from build123d import *

# Parameters (mm, degrees)
SKETCH_R        = 2.1
PAD_DEPTH       = 7
SKETCH001_R     = 2.25
POCKET_DEPTH    = 22.001
POCKET001_DEPTH = 3.5
SKETCH003_R     = 4.3
POCKET002_DEPTH = 5
SKETCH004_R     = 62
SKETCH004_R_2   = 56
POCKET003_DEPTH = 14.001
CHAMFER_SIZE2   = 3
CHAMFER_SIZE    = 5
FILLET_R        = 2.5
FILLET001_R     = 0.5
POCKET004_DEPTH = 4
SKETCH006_R     = 2.1
PAD001_DEPTH    = 0.2


with BuildPart() as part:
    # Sketch → Pad (new body, symmetric)
    with BuildSketch(Plane.XY):
        with BuildLine():
            Line((-8.5, 20), (-8.5, -20))
            Line((-8.5, -20), (5.5, -20))
            Line((5.5, -20), (5.5, -4))
            Line((5.5, -4), (3.887632, -0.941445))
            ThreePointArc((3.538431, 1.865343), (-3.969398, -0.493844), (3.887632, -0.941445))
            Line((6.5, -3.752556), (3.538431, 1.865343))
            Line((6.5, -15), (6.5, -3.752556))
            Line((13.5, -15), (6.5, -15))
            Line((13.5, -2), (13.5, -15))
            Line((5.5, 13.175467), (13.5, -2))
            Line((5.5, 20), (5.5, 13.175467))
            Line((-8.5, 20), (5.5, 20))
        make_face()
        with Locations((0, 14)):
            Circle(SKETCH_R, mode=Mode.SUBTRACT)
        with Locations((0, -14)):
            Circle(SKETCH_R, mode=Mode.SUBTRACT)
    extrude(amount=PAD_DEPTH, both=True)

    # Sketch001 (on Face10 of Pad) → Pocket (cut, through all)
    with BuildSketch(Plane.YZ.offset(13.5)):
        with Locations((-8, 0)):
            Circle(SKETCH001_R)
    extrude(amount=-POCKET_DEPTH, mode=Mode.SUBTRACT)

    # Sketch002 (on Face15 of Pocket) → Pocket001 (cut)
    with BuildSketch(Plane.YZ.offset(13.5)):
        Polygon((-4.5, 2.020726), (-8, 4.041452), (-11.5, 2.020726), (-11.5, -2.020726), (-8, -4.041452), (-4.5, -2.020726), align=None)
    extrude(amount=-POCKET001_DEPTH, mode=Mode.SUBTRACT)

    # Sketch003 (on Face2 of Pocket001) → Pocket002 (cut)
    with BuildSketch(Plane(origin=(-8.5, 0, 0), x_dir=(0, -1, 0), z_dir=(-1, 0, 0))):
        with Locations((8, 0)):
            Circle(SKETCH003_R)
    extrude(amount=-POCKET002_DEPTH, mode=Mode.SUBTRACT)

    # Sketch004 (on Face5 of Pocket002) → Pocket003 (cut, through all)
    with BuildSketch(Plane.XY.offset(7)):
        with Locations((47.5, 0)):
            Circle(SKETCH004_R)
        with Locations((47.5, 0)):
            Circle(SKETCH004_R_2, mode=Mode.SUBTRACT)
    extrude(amount=-POCKET003_DEPTH, mode=Mode.SUBTRACT)

    # Chamfer
    chamfer_edges = [part.edges().sort_by_distance(p)[0] for p in [
        (5.5, -20, 0),
    ]]
    chamfer_side = part.faces().sort_by_distance((5.5, -12.305712, 0))[0]
    chamfer(chamfer_edges, length=CHAMFER_SIZE, length2=CHAMFER_SIZE2, reference=chamfer_side)

    # Fillet
    fillet_edges = [part.edges().sort_by_distance(p)[0] for p in [
        (2.5, -20, 0),
        (-4.806787, -20, 0),
        (13.5, -15, 0),
        (5.5, 20, 0),
        (13.5, -2, 0),
        (5.5, 13.175467, 0),
        (-4.806787, 20, 0),
    ]]
    fillet(fillet_edges, radius=FILLET_R)

    # Fillet001
    fillet001_edges = [part.edges().sort_by_distance(p)[0] for p in [
        (3.887632, -0.941445, 0),
    ]]
    fillet(fillet001_edges, radius=FILLET001_R)

    # Sketch005 (on Face1 of Fillet001) → Pocket004 (cut)
    with BuildSketch(Plane(origin=(0, 0, -7), x_dir=(1, 0, 0), z_dir=(0, 0, -1))):
        Polygon((4.041452, 14), (2.020726, 17.5), (-2.020726, 17.5), (-4.041452, 14), (-2.020726, 10.5), (2.020726, 10.5), align=None)
        Polygon((4.041452, -14), (2.020726, -10.5), (-2.020726, -10.5), (-4.041452, -14), (-2.020726, -17.5), (2.020726, -17.5), align=None)
    pocket004 = extrude(amount=-POCKET004_DEPTH, mode=Mode.SUBTRACT)

    # Mirrored: Pocket004 across XY
    add(pocket004.mirror(Plane.XY), mode=Mode.SUBTRACT)

    # Sketch006 (on Face46 of Mirrored) → Pad001 (join)
    with BuildSketch(Plane(origin=(0, 0, -3), x_dir=(1, 0, 0), z_dir=(0, 0, -1))):
        with Locations((0, 14)):
            Circle(SKETCH006_R)
        with Locations((0, -14)):
            Circle(SKETCH006_R)
    extrude(amount=-PAD001_DEPTH)


solid = part.part
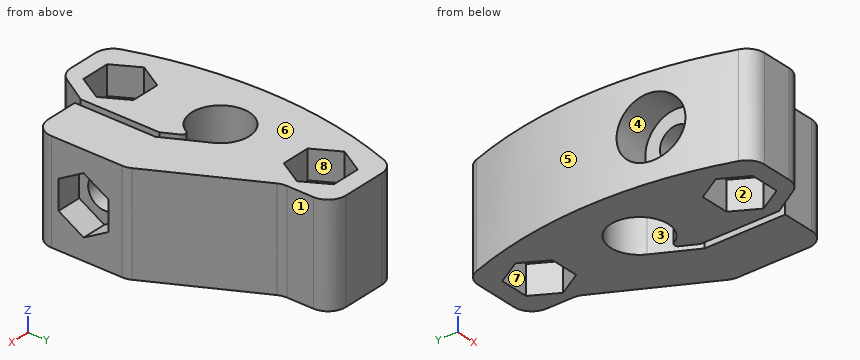
Geometry check sheet. Reference: the model listing, model coordinates, mm. Face numbers are marked on the shaded views. A direction names the side the tool comes from. Coordinates: 2 decimals unless noted, no trailing zeros. Order: outer loops, then holes, each group sorted by start corner. A loop starts at its lowest first (then second) coordinate and runs counter-clockwise, first axis right, second up. Notation, with made-up numbers: (69.25, -24.5) - (108.25, -24.5) arc R26 ccw to (108.25, 3.5) - close; hole circle Ø2 at (-30.75, -3). An arc over 180 degrees is marked (long way). Answer in a Markdown table with one row per item. Add a question column.
1) Set-up check for the marked faces 1, 2, 3 and 4: record each of +Z, -Z, +X, -X, +Y, -Y from which the full face is reachable in a straight line by a thin tool's end or side.
2) Cross-section at B-B, the plane y = 0. Record the cut outline in (x, z), then the cut area to 3 significant figures.
3) Gauge pin test, flat ends, axial feed: P1, Ø5, axis at x = -6, z = 1.5, coming from the +Y side; P2, Ø3.5, axis at x = 0.5, y = -14.5, coming from the -Z side; P3, Ø10.5, axis at x = 0, y = 0, coming from the +Z side; P4, Ø6, axis at x = 9, z = 2, coming from the +Y side. Record the tip position at first contact, or that the pin passes through.
4) Cross-section at A-A, the plane x = 0. State how many separate pieces and enclosed holes the cut face has, then the cut area to 3 significant figures.
5) Cross-section at D-D, the plane x = 7.5. Record the cut outline in (y, z), then the cut area to 3 significant figures.
6) Material ranges on line 1 along Z through (x, y) = (8.4, -8); line 2 along X through (y, z) = (-13.5, -5); line 3 along Y through (x, z) = (0, -1.45), recorded low to high. Write a range as [from, to].
7) Release check for a two-part mould opening along X. For the marked faces 5, 6, 7 and 8 record: +X half, -X half, draft (parallel to the pull), parting line (faces both ways), or undercut.
Check result:
| question | item | result |
|---|---|---|
| 1 | face 1 | +Z, -Z, +X, +Y |
| 1 | face 2 | -Z |
| 1 | face 3 | +Z, -Z |
| 1 | face 4 | -X |
| 2 | outline | (-8.5, -7) - (-4, -7) - (-4, 7) - (-8.5, 7) - close; (4.52, -7) - (12.45, -7) - (12.45, 7) - (4.52, 7) - close |
| 2 | area | 174 mm² |
| 3 | P1 | stops at y = 19.96 |
| 3 | P2 | stops at z = -3 |
| 3 | P3 | stops at z = 7 |
| 3 | P4 | stops at y = 12.23 |
| 4 | separate pieces | 2 |
| 4 | enclosed holes | 1 |
| 4 | area | 271 mm² |
| 5 | outline | (-15, -7) - (9.38, -7) - (9.38, 7) - (-15, 7) - close; hole circle Ø4.5 at (-8, 0) |
| 5 | area | 325 mm² |
| 6 | line 1 | z = [-7, -2.25], [2.25, 7] |
| 6 | line 2 | x = [-6.85, -3.75], [3.75, 5.5], [6.5, 13.29] |
| 6 | line 3 | y = [-20, -16.1], [-11.9, -9.72], [-6.28, -4], [4, 11.9], [16.1, 20] |
| 7 | face 5 | -X half |
| 7 | face 6 | draft |
| 7 | face 7 | undercut |
| 7 | face 8 | undercut |
